```python
from build123d import *

# Parameters (mm, degrees)
SKETCH1_W           = 99
SKETCH1_H           = 202
BOSS_EXTRUDE1_DEPTH = 2
SKETCH2_W           = 97
SKETCH2_H           = 2
BOSS_EXTRUDE2_DEPTH = 82
SKETCH3_W           = 2
SKETCH3_H           = 202
BOSS_EXTRUDE3_DEPTH = 30
FILLET1_R           = 2
SKETCH5_R           = 20
SKETCH5_R_2         = 5.5
CUT_EXTRUDE1_DEPTH  = 41


with BuildPart() as part:
    # Sketch1 → Boss-Extrude1 (new body)
    with BuildSketch(Plane(origin=(0, 0, 0), x_dir=(0, 0, -1), z_dir=(1, 0, 0))):
        with Locations((49.5, 101)):
            Rectangle(SKETCH1_W, SKETCH1_H)
    extrude(amount=BOSS_EXTRUDE1_DEPTH)

    # Sketch2 → Boss-Extrude2 (add)
    with BuildSketch(Plane(origin=(2, 0, 0), x_dir=(0, 0, -1), z_dir=(1, 0, 0))):
        with Locations((48.5, 1)):
            Rectangle(SKETCH2_W, SKETCH2_H)
    extrude(amount=BOSS_EXTRUDE2_DEPTH)

    # Sketch3 → Boss-Extrude3 (add)
    with BuildSketch(Plane(origin=(2, 0, 0), x_dir=(0, 0, -1), z_dir=(1, 0, 0))):
        with Locations((98, 101)):
            Rectangle(SKETCH3_W, SKETCH3_H)
    extrude(amount=BOSS_EXTRUDE3_DEPTH)

    # Fillet1
    fillet1_edges = [part.edges().sort_by_distance(p)[0] for p in [
        (16, 0, -99),
        (0, 0, -49.5),
        (0, 101, -99),
    ]]
    fillet(fillet1_edges, radius=FILLET1_R)

    # Sketch5 → Cut-Extrude1 (cut)
    with BuildSketch(Plane.ZY):
        with Locations((-49.5, 100)):
            Circle(SKETCH5_R)
        with Locations((-24.5, 125)):
            Circle(SKETCH5_R_2)
        with Locations((-74.5, 125)):
            Circle(SKETCH5_R_2)
        with Locations((-24.5, 75)):
            Circle(SKETCH5_R_2)
        with Locations((-74.5, 75)):
            Circle(SKETCH5_R_2)
    extrude(amount=-CUT_EXTRUDE1_DEPTH, mode=Mode.SUBTRACT)


solid = part.part
```
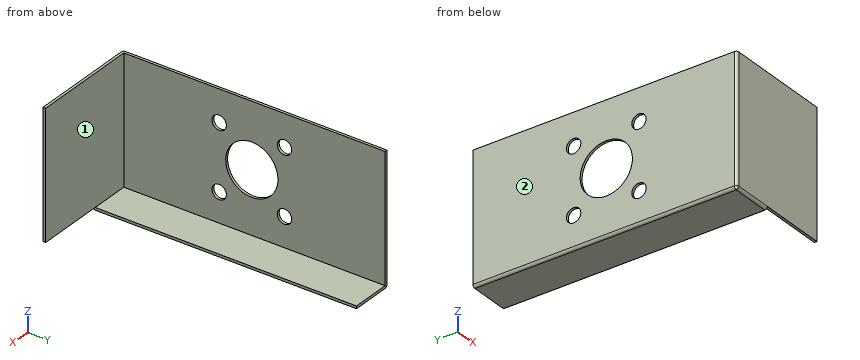
Verification items for the finished model (mm, model axes). Face numbers are marked on the shaded views. A direction names the side the tool comes from. Coordinates: 2 decimals unless noted, no trailing zeros. Write each loop counter-clockwise with the first axis right and the second up, starting at its lowest first coordinate (ties: lowest second). Pieces come first, ordered by that corner, then holes. Notation, with made-up numbers: (-20.5, 43.5) - (1.5, 43.5) arc R22 ccw to (1.5, 63.5) - close; hole circle Ø8 at (49.5, 2). An arc over 180 degrees is marked (long way). Write item = value, one per line.
Q1. Access from +Z, -Z, +X, -X, +Y, -Y to the whole of each face (thin tool, end or side, straight path). Record for the marked faces 1 and 2.
Answer:
face_1 = +Z, +X, +Y
face_2 = +Z, -Z, -X, +Y, -Y
Q2. Material ranges on L1, parallel to Y at x = 1.5, z = -24.5; L2, parallel to Z at x = 20.5, y = 160; L3, parallel to X at y = 13.5, z = -40, recorded low to high. Write a range as from..to.
Answer:
L1 = 0.06..69.5, 80.5..119.5, 130.5..202
L2 = -99..-97
L3 = 0..2
Q3. Cross-section at A-A (z = -49.5). Enter the section's corners in (x, y).
Answer:
outline = (0, 2) arc R2 ccw to (2, 0) - (84, 0) - (84, 2) - (2, 2) - (2, 80) - (0, 80) - close; (0, 120) - (2, 120) - (2, 202) - (0, 202) - close
Q4. Cross-section at C-C (z = -24.5). Enter the section's corners in (x, y), plus the area to 3 significant figures.
Answer:
outline = (0, 2) arc R2 ccw to (2, 0) - (84, 0) - (84, 2) - (2, 2) - (2, 69.5) - (0, 69.5) - close; (0, 80.5) - (2, 80.5) - (2, 119.5) - (0, 119.5) - close; (0, 130.5) - (2, 130.5) - (2, 202) - (0, 202) - close
area = 523 mm²
Q5. Go/stop test with flat-tipped pins: pin 1 Ø12 at (y, z) = (26, -85) entering from +X; pin 2 Ø2 at (x, z) = (39.5, -18.5) entering from +Y; pin 3 Ø9 at (x, y) = (22.5, 73.5) entering from +Z; pin 4 Ø9 at (y, z) = (75, -24.5) entering from -X. Record where each tip stops, or that it passes through.
Answer:
pin_1 = 2
pin_2 = 2
pin_3 = -97
pin_4 = through
Q6. Cross-section at D-D (y = 75). Enter the section's corners in (x, z), plus the area to 3 significant figures.
Answer:
outline = (0, -97) arc R2 ccw to (2, -99) - (32, -99) - (32, -97) - (2, -97) - (2, -80) - (0, -80) - close; (0, -69) - (2, -69) - (2, -30) - (0, -30) - close; (0, -19) - (2, -19) - (2, 0) - (0, 0) - close
area = 213 mm²
Q7. Cross-section at B-B (y = 100). Enter the section's corners in (x, z), plus the area to 3 significant figures.
Answer:
outline = (0, -97) arc R2 ccw to (2, -99) - (32, -99) - (32, -97) - (2, -97) - (2, -69.5) - (0, -69.5) - close; (0, -29.5) - (2, -29.5) - (2, 0) - (0, 0) - close
area = 177 mm²
